Input: part model. Units: mm. Frame: model coordinates. A direction names the side the tool comes from. Coordinates: 2 decimals unless noted, no trailing zeros. Order: outer loops, then holes, each group sorted by start corner. A loop starts at its lowest first (then second) coordinate and runs counter-clockwise, first axis right, second up. Notation, with made-up numbers: (-38.5, -21.5) - (15.5, -21.5) arc R14 cw to (15.5, -12.5) - close; hole circle Ø9 at (53, 12.5). An arc over 180 degrees is marked (long way). Answer as CSV lines item,"result". Start each with the question number.
Item 1: Draft query along X for faces 6 (the flat face through (0, 40, 1)), 7 (the flat face through (41, 91.5, 2)), 8 (the flat face through (-21.59, 88.08, 1.52)). Return one class per face: +X half, -X half, draft (parallel to the pull), parting line (faces both ways), or undercut.
Item 2: Material intervals for line 1 along X through (y, z) = (11.5, 2.05); line 2 along Y through (x, z) = (-11, 1.45); line 3 along Y through (x, z) = (-10.5, 1.4), sorted ascending.
Item 3: Section A-A (x = -29.5). Output: boundary loops of the cut face in (y, z), and give its area (3 significant figures).
Item 4: Access query for faces 1 (the flat face through (38.5, 94, 1)), 2 (the flat face through (19, 81, 1)), 3 (the flat face through (-20, -6, 2)), 4 (the flat face through (-31, -3, 2)), 5 (the flat face through (-33.58, 85.55, 1.52)). Directions: +Z, -Z, +X, -X, +Y, -Y. A direction counts if a zero-diameter tool reaches every point of the face in a straight line with its end or side. Return the directions, or none.
Item 5: Section C-C (y = 82.5). Output: boundary loops of the cut face in (x, z).
Item 6: First-contact query: pin 1 (1 mm diameter, centred on y = 50.5, z = 2, fed in from +X); pin 2 (1.5 mm diameter, centred on x = -43, z = 0.5, fed in from +Y); pin 3 (1 mm diameter, centred on x = -49.5, z = 2, fed in from +Y). Flat tips, straight axial feed; report the tip coordinate or a pass-through.
Item 7: Section B-B (z = 2.4). Output: boundary loops of the cut face in (x, y).
Item 8: Section D-D (x = -54). Output: boundary loops of the cut face in (y, z), and give its area (3 significant figures).
from build123d import *

# Parameters (mm, degrees)
BOSS_EXTRUDE1_DEPTH = 3
CUT_EXTRUDE1_DEPTH  = 125.045354609
SKETCH3_W           = 6
SKETCH3_H           = 6
SKETCH3_W_2         = 22
BOSS_EXTRUDE2_DEPTH = 3


with BuildPart() as part:
    # Sketch1 → Boss-Extrude1 (new body)
    with BuildSketch(Plane.XY):
        Polygon((-78.5, 93), (-78.5, 81), (-40, 81), (-40, 0), (0, 0), (0, 81), (38.5, 81), (38.5, 96), align=None)
    extrude(amount=BOSS_EXTRUDE1_DEPTH)

    # Sketch2 → Cut-Extrude1 (cut, through all)
    with BuildSketch(Plane.XY.offset(3)):
        Polygon((-33.71, 87.02), (-33.448532772, 84.031415906), (-9.539860018, 86.123153732), (-9.801327246, 89.111737826), align=None)
    extrude(amount=-CUT_EXTRUDE1_DEPTH, mode=Mode.SUBTRACT)

    # Sketch3 → Boss-Extrude2 (add, through all)
    with BuildSketch(Plane.XY.offset(3)):
        with Locations((41.5, 88.5)):
            Rectangle(SKETCH3_W, SKETCH3_H)
        with Locations((-20, -3)):
            Rectangle(SKETCH3_W_2, SKETCH3_H)
    extrude(amount=-BOSS_EXTRUDE2_DEPTH)


solid = part.part
Determined:
1,face 6,"+X half"
1,face 7,"draft"
1,face 8,"undercut"
2,line 1,"x = -40 to 0"
2,line 2,"y = -6 to 86, 89.01 to 94.73"
2,line 3,"y = -6 to 86.04, 89.05 to 94.74"
3,outline,"(-6, 0) - (84.38, 0) - (84.38, 3) - (-6, 3) - close; (87.39, 0) - (94.26, 0) - (94.26, 3) - (87.39, 3) - close"
3,area,"292 mm^2"
4,face 1,"+Z, -Z, +X, +Y"
4,face 2,"+Z, -Z, +X, -Y"
4,face 3,"+Z, -Z, +X, -X, -Y"
4,face 4,"+Z, -Z, -X, -Y"
4,face 5,"+Z, -Z"
5,outline,"(-78.5, 0) - (38.5, 0) - (38.5, 3) - (-78.5, 3) - close"
6,pin 1,"stops at x = 0"
6,pin 2,"stops at y = 93.93"
6,pin 3,"stops at y = 93.76"
7,outline,"(-78.5, 81) - (-40, 81) - (-40, 0) - (-31, 0) - (-31, -6) - (-9, -6) - (-9, 0) - (0, 0) - (0, 81) - (38.5, 81) - (38.5, 85.5) - (44.5, 85.5) - (44.5, 91.5) - (38.5, 91.5) - (38.5, 96) - (-78.5, 93) - close; hole (-33.71, 87.02) - (-33.45, 84.03) - (-9.54, 86.12) - (-9.8, 89.11) - close"
8,outline,"(81, 0) - (93.63, 0) - (93.63, 3) - (81, 3) - close"
8,area,"37.9 mm^2"
